Verification items for the finished model (mm, model axes). Give positions to 0.01 mm unless a question says otherwise; leave off trailing zeros. Loops run counter-clockwise (first coordinate to the right, second up) from the corner with the lowest first, then second, coordinate; pieces in that order, holes last. Notation, with made-up numbers: M -2,9 L 5,9 A23 ccw 5,39 Z; hole C 15.5,81 d8. An arc over 180 degrees is marked long. Write each question's results on one line, items separated by ' | '. Start each with the question number.
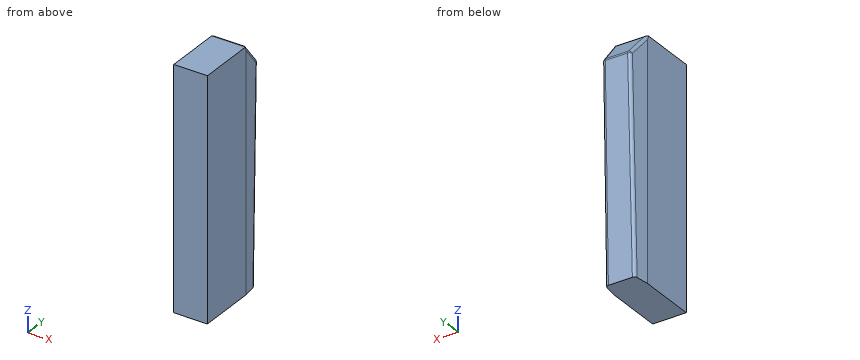
```python
from build123d import *

# Parameters (mm, degrees)
CROQUIS1_W              = 11
CROQUIS1_H              = 78
SALIENTE_EXTRUIR1_DEPTH = 26
CORTAR_EXTRUIR3_DEPTH   = 83.95179323
CORTAR_EXTRUIR6_DEPTH   = 83.95179323
CORTAR_EXTRUIR7_DEPTH   = 83.95179323
REDONDEO4_R             = 1


with BuildPart() as part:
    # Croquis1 → Saliente-Extruir1 (new body)
    with BuildSketch(Plane(origin=(0, 0, 0), x_dir=(1, 0, 0), z_dir=(0, 1, 0))):
        with Locations((5.5, 39)):
            Rectangle(CROQUIS1_W, CROQUIS1_H)
    extrude(amount=SALIENTE_EXTRUIR1_DEPTH)

    # Croquis4 → Cortar-Extruir3 (cut, through all)
    with BuildSketch(Plane.XY):
        Polygon((0, 26), (1, 26), (0, 19), align=None)
        Polygon((10, 26), (11, 26), (11, 19), align=None)
    extrude(amount=-CORTAR_EXTRUIR3_DEPTH, mode=Mode.SUBTRACT)

    # Croquis6 → Cortar-Extruir6 (cut, through all)
    with BuildSketch(Plane.ZY):
        Polygon((0, 19), (0, 26), (-8, 26), align=None)
    extrude(amount=-CORTAR_EXTRUIR6_DEPTH, mode=Mode.SUBTRACT)

    # Croquis8 → Cortar-Extruir7 (cut, through all)
    with BuildSketch(Plane.ZY):
        Polygon((-80, 26), (-6.869978001, 26), (-80, 24), align=None)
    extrude(amount=-CORTAR_EXTRUIR7_DEPTH, mode=Mode.SUBTRACT)

    # Redondeo4
    # the kernel refuses this fillet: 1 mm, written as the material it takes off along each edge
    with BuildSketch(Plane(origin=(1.86153901, 24.959705258, -8.329683982), x_dir=(-0.5677189271234413, -0.022505525063317232, -0.8229147714845281), z_dir=(-0.44431309218949805, 0.8499040291343537, 0.28328257512631844))) as redondeo4_piece_1_section:
        Polygon((-1.655326892, -1.655326892), (1.655326892, -1.655326892), (1.655326892, 1.655326892), (-1.655326892, 1.655326892), align=None)
    redondeo4_piece_1 = extrude(amount=1.655326892, mode=Mode.PRIVATE)
    redondeo4_piece_1 = split(redondeo4_piece_1, bisect_by=Plane(origin=(1.86153901, 24.959705258, -8.329683982), z_dir=(-1, 0, 0)), keep=Keep.TOP, mode=Mode.PRIVATE)
    redondeo4_piece_1 = split(redondeo4_piece_1, bisect_by=Plane(origin=(1.86153901, 24.959705258, -8.329683982), z_dir=(0.09365858115816941, 0.6556100681071857, -0.7492686492653552)), keep=Keep.TOP, mode=Mode.PRIVATE)
    redondeo4_piece_1 = split(redondeo4_piece_1, bisect_by=Plane(origin=(1.86153901, 24.959705258, -8.329683982), z_dir=(0.0039054455429706233, 0.02733811880079436, 0.9996186146503798)), keep=Keep.TOP, mode=Mode.PRIVATE)
    redondeo4_piece_1 = split(redondeo4_piece_1, bisect_by=Plane(origin=(1.86153901, 25.959331496, -8.357022309), z_dir=(0, -0.9996262380814909, 0.027338327290574692)), keep=Keep.TOP, mode=Mode.PRIVATE)
    redondeo4_piece_1 = split(redondeo4_piece_1, bisect_by=Plane(origin=(1.86153901, 25.712281952, -7.671179374), z_dir=(0, -0.7525766947068778, -0.658504607868518)), keep=Keep.TOP, mode=Mode.PRIVATE)
    redondeo4_piece_1 = split(redondeo4_piece_1, bisect_by=Plane(origin=(0.871589516, 25.101126614, -8.329683982), z_dir=(0.9899494936611666, -0.14142135623730953, 0)), keep=Keep.TOP, mode=Mode.PRIVATE)
    redondeo4_piece_1 = redondeo4_piece_1 - Plane(origin=(1.86153901, 24.959705258, -8.329683982), x_dir=(0.44431309218949805, -0.8499040291343537, -0.28328257512631844), z_dir=(-0.5677189271234413, -0.022505525063317232, -0.8229147714845281)) * Sphere(REDONDEO4_R, mode=Mode.PRIVATE)
    add(redondeo4_piece_1, mode=Mode.SUBTRACT)
    with BuildSketch(Plane(origin=(9.13846099, 24.959705258, -8.329683982), x_dir=(-0.5677189271234413, 0.02250552506331723, 0.8229147714845281), z_dir=(0.44431309218949794, 0.8499040291343537, 0.2832825751263184))) as redondeo4_piece_2_section:
        Polygon((-1.655326892, -1.655326892), (1.655326892, -1.655326892), (1.655326892, 1.655326892), (-1.655326892, 1.655326892), align=None)
    redondeo4_piece_2 = extrude(amount=1.655326892, mode=Mode.PRIVATE)
    redondeo4_piece_2 = split(redondeo4_piece_2, bisect_by=Plane(origin=(9.13846099, 24.959705258, -8.329683982), z_dir=(1, 0, 0)), keep=Keep.TOP, mode=Mode.PRIVATE)
    redondeo4_piece_2 = split(redondeo4_piece_2, bisect_by=Plane(origin=(9.13846099, 24.959705258, -8.329683982), z_dir=(-0.09365858115816958, 0.6556100681071857, -0.7492686492653552)), keep=Keep.TOP, mode=Mode.PRIVATE)
    redondeo4_piece_2 = split(redondeo4_piece_2, bisect_by=Plane(origin=(9.13846099, 24.959705258, -8.329683982), z_dir=(-0.0039054455429706303, 0.02733811880079436, 0.9996186146503798)), keep=Keep.TOP, mode=Mode.PRIVATE)
    redondeo4_piece_2 = split(redondeo4_piece_2, bisect_by=Plane(origin=(9.13846099, 25.959331496, -8.357022309), z_dir=(0, -0.9996262380814909, 0.027338327290574692)), keep=Keep.TOP, mode=Mode.PRIVATE)
    redondeo4_piece_2 = split(redondeo4_piece_2, bisect_by=Plane(origin=(9.13846099, 25.712281952, -7.671179374), z_dir=(0, -0.7525766947068778, -0.658504607868518)), keep=Keep.TOP, mode=Mode.PRIVATE)
    redondeo4_piece_2 = split(redondeo4_piece_2, bisect_by=Plane(origin=(10.128410484, 25.101126614, -8.329683982), z_dir=(-0.9899494936611666, -0.14142135623730978, 0)), keep=Keep.TOP, mode=Mode.PRIVATE)
    redondeo4_piece_2 = redondeo4_piece_2 - Plane(origin=(9.13846099, 24.959705258, -8.329683982), x_dir=(-0.44431309218949794, -0.8499040291343537, -0.2832825751263184), z_dir=(-0.5677189271234413, 0.02250552506331723, 0.8229147714845281)) * Sphere(REDONDEO4_R, mode=Mode.PRIVATE)
    add(redondeo4_piece_2, mode=Mode.SUBTRACT)
    with BuildSketch(Plane(origin=(-1.134420566, 19, 0), x_dir=(0, -1, 0), z_dir=(1, 0, 0))) as redondeo4_piece_3:
        with BuildLine():
            CenterArc((REDONDEO4_R * 0.453768226592, REDONDEO4_R), REDONDEO4_R, 221.185925166, 48.814074834)
            Line((-REDONDEO4_R * 0.298808468115, REDONDEO4_R * 0.341495392131), (0, 0))
            Line((0, 0), (REDONDEO4_R * 0.453768226592, 0))
        make_face()
    extrude(amount=13.268841133, mode=Mode.SUBTRACT)
    with BuildSketch(Plane(origin=(0.96681533, 25.767707313, -7.734522643), x_dir=(0.9956043743251828, -0.06167460725908129, 0.07048526543895174), z_dir=(-0.09365858115816941, -0.6556100681071857, 0.7492686492653552)), Plane(origin=(12.052106546, 11.635254179, 8.416852367), x_dir=(-0.9956043743251827, -0.061674607259081395, 0.07048526543895185), z_dir=(-0.09365858115816958, 0.6556100681071857, -0.7492686492653552))) as redondeo4_piece_4:
        with BuildLine():
            CenterArc((REDONDEO4_R * 0.898673913625, -REDONDEO4_R), REDONDEO4_R, 90, 83.890414747)
            Line((-REDONDEO4_R * 0.0956462392286, -REDONDEO4_R * 0.893569583162), (0, 0))
            Line((0, 0), (REDONDEO4_R * 0.898673913625, 0))
        make_face()
    extrude(amount=21.556186859, mode=Mode.SUBTRACT)
    with BuildSketch(Plane(origin=(1.86153901, 25.970032196, -7.965751081), x_dir=(0, -0.6585046078685161, 0.7525766947068797), z_dir=(1, 0, 0))) as redondeo4_piece_5:
        with BuildLine():
            CenterArc((REDONDEO4_R * 0.391417524948, REDONDEO4_R), REDONDEO4_R, 227.247508882, 42.752491118)
            Line((-REDONDEO4_R * 0.287415146966, REDONDEO4_R * 0.265707004295), (0, 0))
            Line((0, 0), (REDONDEO4_R * 0.391417524948, 0))
        make_face()
    extrude(amount=7.27692198, mode=Mode.SUBTRACT)
    with BuildSketch(Plane(origin=(0.994203443, 25.9594241, -8.353636218), x_dir=(-0.14136742020391727, -0.9895719414274202, 0.027615670269893054), z_dir=(-0.0039054455429706233, -0.02733811880079436, -0.9996186146503798)), Plane(origin=(10.286368809, 23.995418339, -80.167528475), x_dir=(0.14136742020391577, -0.9895719414274206, 0.027615670269893058), z_dir=(-0.0039054455429706303, 0.02733811880079436, 0.9996186146503798))) as redondeo4_piece_6:
        with BuildLine():
            CenterArc((REDONDEO4_R * 0.867342181609, -REDONDEO4_R), REDONDEO4_R, 90, 81.872956917)
            Line((-REDONDEO4_R * 0.122614861744, -REDONDEO4_R * 0.85863150168), (0, 0))
            Line((0, 0), (REDONDEO4_R * 0.867342181609, 0))
        make_face()
    extrude(amount=71.841291473, mode=Mode.SUBTRACT)


solid = part.part
```
1. Section check A-A, the plane x = 6. Record the boundary of the cut face in (y, z).
2. Thickness scan on probe 1 along Y at (x, z) = (2, -17); probe 2 along Y at (x, z) = (6, -71.5); probe 3 along Z at (x, y) = (0.5, 19.5). Record the ranges inside material, lowest first.
3. Depth check by flat-ended pin: pin 1 Ø1 at (x, z) = (8.5, -64.5) entering from +Y; pin 2 Ø2 at (x, z) = (9, -40) entering from +Y. Enter the tip coordinate at first touch or a pass-through.
Filled sheet:
1) outline: M 0,-78 L 24.05,-78 L 25.96,-8.36 A1 ccw 25.71,-7.67 L 19.3,-0.34 A1 ccw 18.55,0 L 0,0 Z
2) probe 1: 0 to 25.72 | probe 2: 0 to 24.23 | probe 3: -78 to -0.76
3) pin 1: y = 24.44 | pin 2: y = 25.12
